Check sheet for the modelled part. Datum: model origin and axes. Units: mm. A direction names the side the tool comes from. Round coordinates to 2 decimals unless told otherwise and drop trailing zeros. Order: outer loops, then holes, each group sorted by start corner. A loop starts at its lowest first (then second) coordinate and runs counter-clockwise, first axis right, second up. Notation, with made-up numbers: (-21.75, -22.5) -> (11.25, -22.5) arc R21 ccw to (11.25, 2.5) -> close; hole circle Ø2 at (45.25, 55.5). An arc over 180 degrees is marked (long way). Answer in a Markdown table with one row per item. Add a question column.
1. Depth check by flat-ended pin: P1, Ø4, axis at y = 0.5, z = 3, coming from the +X side; P2, Ø6, axis at x = 2, y = 5, coming from the -Z side; P3, Ø1.5, axis at y = -10.5, z = 2, coming from the +X side. Enter the tip coordinate at first touch or a pass-through.
2. Sectioned sample at A-A, the plane y = 2.5. Record the boundary of the cut face in (x, z).
3. Material ranges on L1, parallel to Y at x = 4.75, z = 2.25; L2, parallel to X at y = 4, z = -0.25; L3, parallel to Y at x = -0.5, z = 4.75, recorded low to high. Write a range as from..to.
4. Draft check along Y on faces 3 (the cylindrical face through (-1.38, 13.02, -0.44)), 4 (the flat face through (0, 15.9, 0)), 5 (the cylindrical face through (-1.38, -12.98, -0.44)), 6 (the cylindrical face through (-1.812, 15.108, -0.571)). Enter one of: +Y half, -Y half, draft (parallel to the pull), parting line (faces both ways), or undercut.
5. Access from +Z, -Z, +X, -X, +Y, -Y to the whole of each face (thin tool, end or side, straight path). Record for faces 1 (the cylindrical face through (-1.812, -15.092, -0.571)), 2 (the flat face through (0, -15.9, 0)).
6. Sectioned sample at B-B, the plane y = 10. Record the boundary of the cut face in (x, z), then the cut area to 3 significant figures.
```python
from build123d import *

# Parameters (mm, degrees)
CONG_1_R = 5
CONG_2_R = 0.2


with BuildPart() as part:
    # Esquisse1 → Révolution1 (revolve)
    with BuildSketch(Plane.XY, mode=Mode.PRIVATE) as r_volution1_sk:
        Polygon((0, 15.9), (0, -15.9), (1.9, -15.9), (1.9, -14.3), (1.45, -14.3), (1.45, -11.7), (7, 0), (1.45, 11.7), (1.45, 14.3), (1.9, 14.3), (1.9, 15.9), align=None)
    revolve(r_volution1_sk.sketch.rotate(Axis((0, 15.9, 0), (0, -1, 0)), 180), axis=Axis((0, 15.9, 0), (0, -1, 0)))  # turned: the seam where the file's is

    # Congé1
    cong_1_edges = [part.edges().sort_by_distance(p)[0] for p in [
        (7, 0, 0),
    ]]
    fillet(cong_1_edges, radius=CONG_1_R)

    # Congé2
    cong_2_edges = [part.edges().sort_by_distance(p)[0] for p in [
        (1.9, -14.3, 0),
        (1.9, 14.3, 0),
        (1.9, 15.9, 0),
        (1.9, -15.9, 0),
    ]]
    fillet(cong_2_edges, radius=CONG_2_R)


solid = part.part
```
Answer key:
| question | item | result |
|---|---|---|
| 1 | P1 | stops at x = 6.38 |
| 1 | P2 | stops at z = -5.89 |
| 1 | P3 | stops at x = 1.74 |
| 2 | outline | circle Ø11.63 at (0, 0) |
| 3 | L1 | y = -3.68..3.68 |
| 3 | L2 | x = -5.1..5.1 |
| 3 | L3 | y = -4.69..4.69 |
| 4 | face 3 | undercut |
| 4 | face 4 | +Y half |
| 4 | face 5 | undercut |
| 4 | face 6 | draft |
| 5 | face 1 | -Y |
| 5 | face 2 | +Z, -Z, +X, -X, -Y |
| 6 | outline | circle Ø4.51 at (0, 0) |
| 6 | area | 16.0 mm² |
